Can you work these out from the model? Positions are in its coordinate system, mm. A direction names the side the tool comes from. Give positions to 0.01 mm unless a question says otherwise; leave off trailing zeros. Loops run counter-clockwise (first coordinate to the right, second up) from the corner with the lowest first, then second, coordinate; pieces in that order, holes last. Notation, with made-up numbers: M 0.5,74 L 24.5,74 A25 ccw 24.5,103 Z; hole C 86,65.25 d1. An arc over 180 degrees is marked long. Use CSV: the item, a comma, the result in double quotes.
from build123d import *

# Parameters (mm, degrees)
SKETCH1_W                        = 50.8
SKETCH1_H                        = 25.4
SKETCH1_W_2                      = 44.45
SKETCH1_H_2                      = 19.05
BOSS_EXTRUDE1_DEPTH              = 728.3704
CUT_EXTRUDE1_DEPTH               = 730.255620202
CUT_EXTRUDE2_DEPTH               = 552.395616702
CUT_EXTRUDE3_DEPTH               = 735.841052167
F_13_64_0_20313_DIAMETER_HOLE1_D = 5.159502
F_13_64_0_20313_DIAMETER_HOLE2_D = 5.159502


with BuildPart() as part:
    # Sketch1 → Boss-Extrude1 (new body)
    with BuildSketch(Plane(origin=(0, 0, 0), x_dir=(1, 0, 0), z_dir=(0, 1, 0))):
        Rectangle(SKETCH1_W, SKETCH1_H)
        Rectangle(SKETCH1_W_2, SKETCH1_H_2, mode=Mode.SUBTRACT)
    extrude(amount=BOSS_EXTRUDE1_DEPTH)

    # Sketch2 → Cut-Extrude1 (cut, through all)
    with BuildSketch(Plane.XY.offset(12.7)):
        Polygon((-25.4, 677.5704), (25.4, 728.3704), (-25.4, 728.3704), align=None)
        Polygon((-11.4046, 0), (-25.4, 13.9954), (-25.4, 0), align=None)
        Polygon((-11.4046, 0), (25.4, 36.8046), (25.4, 0), align=None)
    extrude(amount=-CUT_EXTRUDE1_DEPTH, mode=Mode.SUBTRACT)

    # Sketch3 → Cut-Extrude2 (cut, through all)
    with BuildSketch(Plane(origin=(376.8852, 376.8852, 0), x_dir=(0, 0, -1), z_dir=(0.7071067811865417, 0.7071067811865535, 0))):
        Polygon((-12.7, 497.075136813), (12.7, 488.822176529), (12.7, 497.075136813), align=None)
    extrude(amount=-CUT_EXTRUDE2_DEPTH, mode=Mode.SUBTRACT)

    # Sketch4 → Cut-Extrude3 (cut, through all)
    with BuildSketch(Plane(origin=(-5.7023, -5.7023, 0), x_dir=(0, 0, 1), z_dir=(-0.7071067811865477, -0.7071067811865475, 0))):
        Polygon((-12.7, 8.064269997), (12.7, 16.317230281), (12.7, 8.064269997), align=None)
    extrude(amount=-CUT_EXTRUDE3_DEPTH, mode=Mode.SUBTRACT)

    # 13/64 (0.20313) Diameter Hole1 (through all)
    with Locations(Plane(origin=(0, 0, -12.7), x_dir=(-1, 0, 0), z_dir=(0, 0, -1))):
        with Locations((0, 623.07659026), (0, 648.47659026), (14.2367, 282.194), (14.2367, 136.398)):
            Hole(F_13_64_0_20313_DIAMETER_HOLE1_D / 2)

    # 13/64 (0.20313) Diameter Hole2 (through all)
    with Locations(Plane.XY.offset(12.7)):
        with Locations((0, 106.89437358), (0, 81.49437358)):
            Hole(F_13_64_0_20313_DIAMETER_HOLE2_D / 2)


solid = part.part
Q1. I want a section at B-B, the plane x = 13. Please give me the cut outline in (y, z) (3 decimals).
Model answer:
outline,"M 24.405,-12.7 L 704.299,-12.7 L 705.758,-9.525 L 25.864,-9.525 Z; M 34.617,9.525 L 714.511,9.525 L 715.97,12.7 L 36.076,12.7 Z"
Q2. For faces 4 (the flat face through (-22.225, 340, 0)), 5 (the flat face through (6.11, 28.08, 10.29)), which set-ups out of +Z, -Z, +X, -X, +Y, -Y let a thin tool reach every point of the face, with its end or its side?
Model answer:
face 4,"+Y, -Y"
face 5,"+Z, +X, -Y"
Q3. I want a section at C-C, the plane z = -1. Please give me the cut outline in (x, y) (3 decimals), then the cut area to 3 significant figures.
Model answer:
outline,"M -25.4,13.995 L -22.225,10.82 L -22.225,674.45 L -25.4,671.275 Z; M 22.225,39.006 L 25.4,42.181 L 25.4,722.075 L 22.225,718.9 Z"
area,"4,260 mm2"
Q4. I want a section at A-A, the plane y = 146.5. Please give me the cut outline in (x, z) (3 decimals).
Model answer:
outline,"M -25.4,-12.7 L 25.4,-12.7 L 25.4,12.7 L -25.4,12.7 Z; hole M -22.225,-9.525 L 22.225,-9.525 L 22.225,9.525 L -22.225,9.525 Z"
Q5. If we mould it in two halves opening along Z, with no side actions, what happens to faces 1 (the flat face through (0, 359, 9.525)), 2 (the flat face through (-25.4, 341, 0)), 3 (the flat face through (-4.36, 697.56, 10.41))? For each: released by +Z, released by -Z, zero draft, split by the parting line, or undercut.
Model answer:
face 1,"undercut"
face 2,"zero draft"
face 3,"released by -Z"
Q6. Please list where these lines run through material, in increasing order: L1, parallel to Z at x = 13, y = 660 (3 decimals); L2, parallel to X at y = 371, z = -0.25 (3 decimals); L3, parallel to Y at x = 0, z = -11.15. Write a range as from..to.
Model answer:
L1,"-12.7..-9.525, 9.525..12.7"
L2,"-25.4..-22.225, 22.225..25.4"
L3,"12.12..78.91, 84.07..104.31, 109.47..620.5, 625.66..645.9, 651.06..692.01"
